Work out the finished part from the listing and answer in its coordinate system (mm). Face numbers are marked on the shaded views. Round coordinates to 2 decimals unless told otherwise and drop trailing zeros. Write each loop counter-clockwise with the first axis right and the second up, starting at its lowest first coordinate (ties: lowest second). Pieces come first, ordered by that corner, then holes.
1. Find section C-C (z = 29.5). Write down the section's boundary in (x, y).
2. Determine the mould class of the marked faces 1 and 2 for opening direction X: pulls with the +X half, pulls with the -X half, needs draft (parallel to the pull), parting line crosses it, or undercut.
3. Straight lines are drawn through the part: probe 1 along Y at (x, z) = (0, 30); probe 2 along X at (y, z) = (6.75, 30.5); probe 3 along Z at (x, y) = (0.25, -0.25) (3 decimals). For each, find the intervals that lie inside material, in ascending order.
4. Find section D-D (z = 55.5). Write down the section's boundary in (x, y).
5. Find section A-A (y = 0). Write down the section's boundary in (x, z), and give its area (3 significant figures).
6. Flat-ended cylindrical pins translate along their axes: pin 1 Ø8 at (y, z) = (-8, 52) entering from -X; pin 2 Ø5 at (y, z) = (-5.5, 35.5) entering from -X; pin 3 Ø3 at (x, z) = (9, 7.5) entering from -Y. Find the tip coordinate at first contact, or state that the pin passes through.
```python
from build123d import *

# Parameters (mm, degrees)
SKETCH_1_R               = 12.5
EXTRUDE_1_DEPTH          = 62.5
FILLET_1_R               = 12.5
CUT_EXTRUDE_1_DEPTH      = 65.951905284
CUT_EXTRUDE_1_DEPTH_BACK = 45
SKETCH_2_R               = 10
SKETCH_3_R               = 10.5
CUT_EXTRUDE_2_DEPTH      = 5


with BuildPart() as part:
    # 草图1 → 凸台-拉伸1 (new body)
    with BuildSketch(Plane.XY):
        Circle(SKETCH_1_R)
    extrude(amount=EXTRUDE_1_DEPTH)

    # 圆角1
    fillet_1_edges = [part.edges().sort_by_distance(p)[0] for p in [
        (-12.5, 0, 62.5),
    ]]
    fillet(fillet_1_edges, radius=FILLET_1_R)

    # 草图2 → 切除-拉伸1 (cut, two sides: drawn at the far end of the back side and taken through both)
    with BuildSketch(Plane(origin=(0, 0, 0), x_dir=(-1, 0, 0), z_dir=(0, 0, -1)).offset(-CUT_EXTRUDE_1_DEPTH_BACK)):
        with Locations(Location((0, 0, 0), (0, 0, 180))):
            Circle(SKETCH_2_R)
    extrude(amount=CUT_EXTRUDE_1_DEPTH + CUT_EXTRUDE_1_DEPTH_BACK, mode=Mode.SUBTRACT)

    # 草图3 → 切除-拉伸2 (cut)
    with BuildSketch(Plane(origin=(0, 0, 45), x_dir=(-1, 0, 0), z_dir=(0, 0, -1))):
        Circle(SKETCH_3_R)
    extrude(amount=-CUT_EXTRUDE_2_DEPTH, mode=Mode.SUBTRACT)


solid = part.part
```
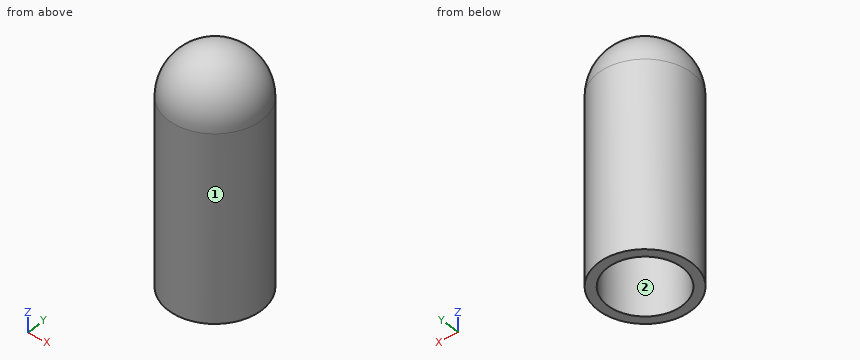
Worked answers:
1. outline: circle Ø25 at (0, 0); hole circle Ø20 at (0, 0)
2. face 1: parting line crosses it
2. face 2: undercut
3. probe 1: y = -12.5 to -10, 10 to 12.5
3. probe 2: x = -10.52 to -7.38, 7.38 to 10.52
3. probe 3: z = 50 to 62.495
4. outline: circle Ø22.45 at (0, 0)
5. outline: (-12.5, 0) - (-10, 0) - (-10, 45) - (-10.5, 45) - (-10.5, 50) - (10.5, 50) - (10.5, 45) - (10, 45) - (10, 0) - (12.5, 0) - (12.5, 50) arc R12.5 ccw to (-12.5, 50) - close
5. area: 490 mm2
6. pin 1: stops at x = -11.76
6. pin 2: stops at x = -12.13
6. pin 3: stops at y = -10
